Could you check a few things on this model? Use its own coordinates, in mm. Round coordinates to 2 decimals unless told otherwise and drop trailing zeros. Loops run counter-clockwise (first coordinate to the right, second up) from the corner with the lowest first, then second, coordinate; pieces in that order, holes last. Notation, with made-up numbers: M -31,61.5 L 26,61.5 A22 cw 26,78.5 Z; hole C 28.25,34.25 d10. An arc over 180 degrees is marked long. One line per item, written item: value. Start each with the question number.
Q1. Please list where these lines run through material, in increasing order: line 1 along Z through (x, y) = (-48.5, -377.5); line 2 along X through (y, z) = (-757.5, 22.5); line 3 along Y through (x, z) = (-61, 2).
Q2. I'm going to push a flat-ended pin straight in: pin 1 Ø12 at (x, z) = (-56.5, 8) entering from +Y. Where does the tip first touch, or does it pass through?
Q3. Imagine slicing it at C-C (x = -53). Please give me the cut outline in (y, z), then the cut area to 3 significant figures.
Q4. Imagine slicing it at B-B (y = -933). Please give me the cut outline in (x, z), then the cut area to 3 significant figures.
Q5. Imagine slicing it at A-A (z = 19.5). Please give me the cut outline in (x, y), then the cut area to 3 significant figures.
from build123d import *

# Parameters (mm, degrees)
F0_W     = 31.75
F0_H     = 31.75
F0_W_2   = 27.5336
F0_H_2   = 27.5336
F1_DEPTH = 2438.4
F3_DEPTH = 76.2


with BuildPart() as f1:
    # F0 (on Front) → F1 (new body)
    with BuildSketch(Plane.XZ):
        with Locations((-48.296367, 16.120737)):
            Rectangle(F0_W, F0_H)
        with Locations((-48.296367, 16.120737)):
            Rectangle(F0_W_2, F0_H_2, mode=Mode.SUBTRACT)
    extrude(amount=F1_DEPTH)

    # F2 (on face) → F3 (cut)
    with BuildSketch(Plane.XY.offset(31.995737)):
        Polygon((-32.421367, 0), (-64.171367, 0), (-32.421367, -31.75), align=None)
        Polygon((-32.421367, -2406.65), (-64.171367, -2438.4), (-32.421367, -2438.4), align=None)
    extrude(amount=-F3_DEPTH, mode=Mode.SUBTRACT)


solid = f1.part
Report:
1. line 1: z = 0.25 to 2.35, 29.89 to 32
1. line 2: x = -64.17 to -62.06, -34.53 to -32.42
1. line 3: y = -2435.23 to -3.17
2. pin 1: stops at y = -1.67
3. outline: M -2427.23,0.25 L -11.17,0.25 L -11.17,2.35 L -2427.23,2.35 Z; M -2427.23,29.89 L -11.17,29.89 L -11.17,32 L -2427.23,32 Z
3. area: 10,200 mm²
4. outline: M -64.17,0.25 L -32.42,0.25 L -32.42,32 L -64.17,32 Z; hole M -62.06,2.35 L -34.53,2.35 L -34.53,29.89 L -62.06,29.89 Z
4. area: 250 mm²
5. outline: M -64.17,-2438.4 L -62.06,-2436.29 L -62.06,-2.11 L -64.17,0 Z; M -34.53,-2408.76 L -32.42,-2406.65 L -32.42,-31.75 L -34.53,-29.64 Z
5. area: 10,100 mm²
